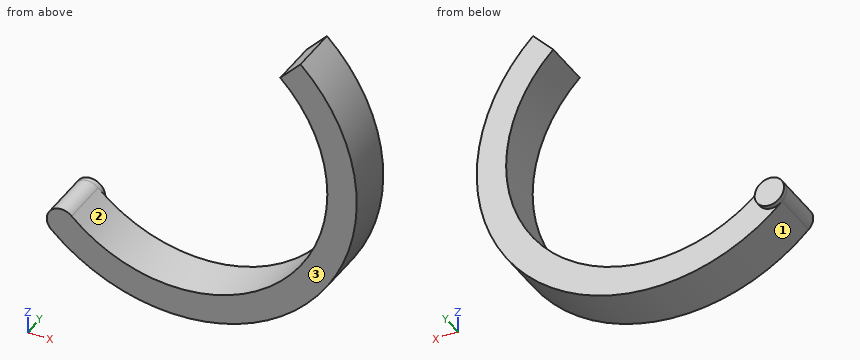
from build123d import *

# Parameters (mm, degrees)
BOSS_EXTRUDE8_DEPTH     = 10
SKETCH17_R              = 3
BOSS_EXTRUDE9_DEPTH     = 1
CUT_EXTRUDE3_DEPTH      = 48
CUT_EXTRUDE3_DEPTH_BACK = 52


with BuildPart() as part:
    # Sketch15 → Boss-Extrude8 (new body)
    with BuildSketch(Plane(origin=(0, 0, 0), x_dir=(1, 0, 0), z_dir=(0, 1, 0))):
        with BuildLine():
            ThreePointArc((48.786503152, -51.330803164), (50.112545273, 0.848485663), (-2.066743554, 2.174527784))
            ThreePointArc((-2.066743554, 2.174527784), (-2.174527784, -2.066743554), (2.066743554, -2.174527784))
            ThreePointArc((2.066743554, -2.174527784), (45.763489705, -3.285001446), (44.653016043, -46.981747597))
            ThreePointArc((44.653016043, -46.981747597), (44.545231814, -51.223018935), (48.786503152, -51.330803164))
        make_face()
    extrude(amount=BOSS_EXTRUDE8_DEPTH)

    # Sketch17 → Boss-Extrude9 (add)
    with BuildSketch(Plane(origin=(0, 10, 0), x_dir=(1, 0, 0), z_dir=(0, 1, 0))):
        with Locations(Location((0, 0, 0), (0, 0, 133.544244871))):
            Circle(SKETCH17_R)
    extrude(amount=BOSS_EXTRUDE9_DEPTH)

    # Sketch18 → Cut-Extrude3 (cut, two sides: drawn at the far end of the back side and taken through both)
    with BuildSketch(Plane(origin=(0, 10, 0), x_dir=(1, 0, 0), z_dir=(0, 1, 0)).offset(-CUT_EXTRUDE3_DEPTH_BACK)):
        with BuildLine():
            Line((44.653016043, -46.981747597), (48.786503152, -51.330803164))
            ThreePointArc((48.786503152, -51.330803164), (46.643544638, -52.155307104), (44.545231814, -51.223018935))
            ThreePointArc((44.545231814, -51.223018935), (43.720727874, -49.080060421), (44.653016043, -46.981747597))
        make_face()
    extrude(amount=CUT_EXTRUDE3_DEPTH + CUT_EXTRUDE3_DEPTH_BACK, mode=Mode.SUBTRACT)


solid = part.part
Model file for the job. Use its own axes, mm. Face numbers are marked on the shaded views. Give positions to 0.01 mm unless a question says otherwise; leave off trailing zeros. Loops run counter-clockwise (first coordinate to the right, second up) from the corner with the lowest first, then second, coordinate; pieces in that order, holes last. Notation, with made-up numbers: (65.25, 63) -> (106.25, 63) arc R11 cw to (106.25, 74) -> close; hole circle Ø10 at (58, 11). An arc over 180 degrees is marked (long way). Use a Markdown table: item, result. Add a question column.
(1) Slice it at D-D on z = 38.5. List the corners of the cut face in (x, y), and give its area (3 significant figures).
(2) Wall check: line 1 along Y through (x, z) = (54.5, 37); line 2 along X through (y, z) = (3.5, 2.5); line 3 along Z through (x, y) = (23, 0.5). Give the ranges that are in metal, low to high.
(3) Slice it at B-B on x = 0. List the corners of the cut face in (y, z).
(4) Drop flat-ended pins along their axis: pin 1 Ø5 at (y, z) = (6.5, 13.5) entering from -X; pin 2 Ø1.5 at (x, y) = (50.5, 7.5) entering from +Z; pin 3 Ø1.5 at (x, y) = (36.5, 4) entering from +Z. Give the stop position or say it passes through.
(5) Slice it at C-C on y = 2. List the corners of the cut face in (x, z), and give its area (3 significant figures).
(6) Slice it at A-A on z = 0. List the corners of the cut face in (x, y), and give its area (3 significant figures).
(7) Mould opens along Z. For the marked faces 1, 2 and 3 say: +Z half, -Z half, draft (parallel to the pull), parting line (faces both ways), or undercut.
Filled sheet:
| question | item | result |
|---|---|---|
| 1 | outline | (50.96, 0) -> (57.54, 0) -> (57.54, 10) -> (50.96, 10) -> close |
| 1 | area | 65.9 mm2 |
| 2 | line 1 | 0 to 10 |
| 2 | line 2 | -1.66 to 1.66, 44.99 to 52.94 |
| 2 | line 3 | -12.33 to -6.33 |
| 3 | outline | (0, -4) -> (10, -4) -> (10, -3) -> (11, -3) -> (11, 3) -> (0, 3) -> close |
| 4 | pin 1 | x = 51.13 |
| 4 | pin 2 | z = 50.38 |
| 4 | pin 3 | z = -3.03 |
| 5 | outline | (-2.07, -2.17) arc R36.91 ccw to (48.79, 51.33) -> (44.65, 46.98) arc R30.91 cw to (2.07, 2.17) arc R3 ccw to start |
| 5 | area | 653 mm2 |
| 6 | outline | (-3, 0) -> (4.62, 0) -> (4.62, 10) -> (3, 10) -> (3, 11) -> (-3, 11) -> close; (42.1, 0) -> (50.89, 0) -> (50.89, 10) -> (42.1, 10) -> close |
| 6 | area | 170 mm2 |
| 7 | face 1 | parting line |
| 7 | face 2 | undercut |
| 7 | face 3 | draft |
